from build123d import *

# Parameters (mm, degrees)
F0_W     = 1500
F0_H     = 1300
F1_DEPTH = 150
F2_W     = 1480
F2_H     = 1280
F3_DEPTH = 130
F4_W     = 1700
F4_H     = 1500
F4_W_2   = 1480
F4_H_2   = 1280
F5_DEPTH = 10
F6_R     = 7.5
F7_DEPTH = 20.001
F8_W     = 10
F8_H     = 203.1123805046
F9_DEPTH = 100


with BuildPart() as f1:
    # F0 (on Top) → F1 (new body)
    with BuildSketch(Plane.XY):
        Rectangle(F0_W, F0_H)
    extrude(amount=F1_DEPTH)

    # F2 (on face) → F3 (cut)
    with BuildSketch(Plane.XY.offset(150)):
        Rectangle(F2_W, F2_H)
    extrude(amount=-F3_DEPTH, mode=Mode.SUBTRACT)

    # F4 (on face) → F5 (join)
    with BuildSketch(Plane.XY.offset(150)):
        Rectangle(F4_W, F4_H)
        Rectangle(F4_W_2, F4_H_2, mode=Mode.SUBTRACT)
    extrude(amount=F5_DEPTH)

    # F6 (on face) → F7 (cut, through all)
    with BuildSketch(Plane.XY.offset(20)):
        with Locations((0, 576.8876194954)):
            Circle(F6_R)
        with Locations((-484.1082007155, -261.6123805046)):
            Circle(F6_R)
        with Locations((484.1082007155, -261.6123805046)):
            Circle(F6_R)
        with Locations((-92, 416.9192598449)):
            Circle(F6_R)
        with Locations((92, 416.9192598449)):
            Circle(F6_R)
        with Locations((-127, 356.8787698224)):
            Circle(F6_R)
        with Locations((127, 356.8787698224)):
            Circle(F6_R)
        with Locations((-230.0749478413, -261.5931819487)):
            Circle(F6_R)
        with Locations((-357.0749478413, -41.6227293875)):
            Circle(F6_R)
        with Locations((-299.5715374564, -261.3025378275)):
            Circle(F6_R)
        with Locations((-391.5715374564, -101.9538635312)):
            Circle(F6_R)
        with Locations((391.5715374564, -101.9538635312)):
            Circle(F6_R)
        with Locations((299.5715374564, -261.3025378275)):
            Circle(F6_R)
        with Locations((230.0749478413, -261.5931819487)):
            Circle(F6_R)
        with Locations((357.0749478413, -41.6227293875)):
            Circle(F6_R)
        with Locations((0, 376.8876194954)):
            Circle(F6_R)
        with Locations((310.9031199586, -161.6123805046)):
            Circle(F6_R)
        with Locations((-310.9031199586, -161.6123805046)):
            Circle(F6_R)
    extrude(amount=-F7_DEPTH, mode=Mode.SUBTRACT)

    # F8 (on face) → F9 (join)
    with BuildSketch(Plane.XY.offset(20)):
        with Locations((-286.2588901058, 538.4438097477)):
            Rectangle(F8_W, F8_H)
        Polygon((-503.4940892386, 51.9649633672), (-281.2588901058, 436.8876194954), (-291.2588901058, 436.8876194954), (-359.9470881013, 317.9161706869), (-365.0381898631, 309.0981237688), (-508.4940892386, 60.6252174051), (-684.3945705787, -40.9309728472), (-679.3945705787, -49.5912268851), align=None)
        Polygon((-365.0381898631, 309.0981237688), (-359.9470881013, 317.9161706869), (-722.3309758605, 631.329262803), (-725.6017355252, 627.5474469407), (-728.8724951898, 623.7656310784), align=None)
        with Locations((286.2588901058, 538.4438097477)):
            Rectangle(F8_W, F8_H)
        Polygon((359.9470881013, 317.9161706869), (291.2588901058, 436.8876194954), (281.2588901058, 436.8876194954), (503.4940892386, 51.9649633672), (508.4940892386, 60.6252174051), (365.0381898631, 309.0981237688), align=None)
        Polygon((722.3309758605, 631.329262803), (359.9470881013, 317.9161706869), (365.0381898631, 309.0981237688), (728.8724951898, 623.7656310784), (725.6017355252, 627.5474469407), align=None)
        Polygon((508.4940892386, 60.6252174051), (503.4940892386, 51.9649633672), (679.3945705787, -49.5912268851), (684.3945705787, -40.9309728472), align=None)
        Polygon((217.2351991328, -443.8499784143), (393.1356804729, -545.4061686666), (398.1356804729, -536.7459146288), (222.2351991328, -435.1897243764), (0, -435.1897243764), (-222.2351991328, -435.1897243764), (-398.1356804729, -536.7459146288), (-393.1356804729, -545.4061686666), (-217.2351991328, -443.8499784143), (0, -443.8499784143), align=None)
        Polygon((-344.6060815022, -640), (-740, 44.842355842), (-748.4989762306, 39.9354696274), (-487.5375583846, -412.0629648972), (-480.1509961227, -424.856866028), (-353.1050577328, -644.9068862146), align=None)
        Polygon((-480.1509961227, -424.856866028), (-487.5375583846, -412.0629648972), (-730.4277149046, -622.1301272929), (-725.6822450561, -627.6170768052), (-720.9367752075, -633.1040263176), align=None)
        Polygon((748.4989762306, 39.9354696274), (740, 44.842355842), (344.6060815022, -640), (353.1050577328, -644.9068862146), (480.1509961227, -424.856866028), (487.5375583846, -412.0629648972), align=None)
        Polygon((730.4277149046, -622.1301272929), (487.5375583846, -412.0629648972), (480.1509961227, -424.856866028), (720.9367752075, -633.1040263176), (725.6822450561, -627.6170768052), align=None)
    extrude(amount=F9_DEPTH)


solid = f1.part
Build history of the part. All positions in model axes, mm. A direction names the side the tool comes from. Round coordinates to 2 decimals unless told otherwise and drop trailing zeros. Write each loop counter-clockwise with the first axis right and the second up, starting at its lowest first coordinate (ties: lowest second). Pieces come first, ordered by that corner, then holes. Notation, with made-up numbers: M -4,29.25 L 17,29.25 A17 ccw 17,41.25 Z; hole C 44,46 d6. An arc over 180 degrees is marked long. Answer in a Markdown table with one row per item.
1. Saw through at D-D (y = 518). List the corners of the cut face in (x, z), and give its area (3 significant figures).
Geometry check:
| item | result |
|---|---|
| outline | M -850,150 L -750,150 L -750,0 L 750,0 L 750,150 L 850,150 L 850,160 L 740,160 L 740,20 L 606.58,20 L 606.58,120 L 591.29,120 L 591.29,20 L 291.26,20 L 291.26,120 L 281.26,120 L 281.26,20 L -281.26,20 L -281.26,120 L -291.26,120 L -291.26,20 L -591.29,20 L -591.29,120 L -606.58,120 L -606.58,20 L -740,20 L -740,160 L -850,160 Z |
| area | 39,900 mm2 |
2. Saw through at B-B (y = -213.5). List the corners of the cut face in (x, z).
Geometry check:
| item | result |
|---|---|
| outline | M -850,150 L -750,150 L -750,0 L 750,0 L 750,150 L 850,150 L 850,160 L 740,160 L 740,20 L 602.18,20 L 602.18,120 L 590.85,120 L 590.85,20 L -590.85,20 L -590.85,120 L -602.18,120 L -602.18,20 L -740,20 L -740,160 L -850,160 Z |
3. Mould opens along Y. For faces 1 (the face through (-4, 670, 150)), 2 (the face through (-418.914, -530.922, 69.3)) say: +Y half, -Y half, draft (parallel to the pull), parting line (faces both ways), or undercut.
Geometry check:
| item | result |
|---|---|
| face 1 | draft |
| face 2 | undercut |
4. Which spindle directions (+Z, -Z, +X, -X, +Y, -Y) get a long thin tool onto all of the face, cutting with end or side? Do faces 3 (the face through (-10, 9, 0)), 4 (the face through (438, 373, 120)). Say none if no direction does.
Geometry check:
| item | result |
|---|---|
| face 3 | -Z, +X, -X, +Y, -Y |
| face 4 | +Z |
5. Probe L1, parallel to Y at x = -69, z = 44.5; L2, parallel to Y at x = -127, z = 12.25; L3, parallel to Y at x = 92, z = 10. List the from-to ranges inside material, lowest first. Write a range as [from, to].
Geometry check:
| item | result |
|---|---|
| L1 | [-650, -640], [-443.85, -435.19], [640, 650] |
| L2 | [-650, 349.38], [364.38, 650] |
| L3 | [-650, 409.42], [424.42, 650] |
6. Flat gauge pins, fed straight in: P1, Ø10, axis at x = -603, z = 141.5, coming from the -Y side; P2, Ø6, axis at x = -539, z = 91, coming from the +Y side; P3, Ø12, axis at x = -391.57, y = -101.95, coming from the -Z side; P4, Ø2, axis at y = -0.5, z = 57, coming from the +X side. Where does each tip first touch, or does it go through?
Geometry check:
| item | result |
|---|---|
| P1 | y = -650 |
| P2 | y = 650 |
| P3 | through |
| P4 | x = 750 |
7. Saw through at A-A (z = 68). State how many separate pieces and enclosed holes the cut face has, and give its area (3 significant figures).
Geometry check:
| item | result |
|---|---|
| separate pieces | 2 |
| enclosed holes | 3 |
| area | 113,000 mm2 |
8. Saw through at C-C (x = -450.5). List the corners of the cut face in (y, z).
Geometry check:
| item | result |
|---|---|
| outline | M -750,150 L -650,150 L -650,0 L 650,0 L 650,150 L 750,150 L 750,160 L 640,160 L 640,20 L 396.23,20 L 396.23,120 L 383.01,120 L 383.01,20 L 161.07,20 L 161.07,120 L 143.75,120 L 143.75,20 L -456.59,20 L -456.59,120 L -476.21,120 L -476.21,20 L -640,20 L -640,160 L -750,160 Z |
